For this review, take the finished solid that the model builds, in its own axes (mm). A direction names the side the tool comes from. Give positions to 0.01 mm unless a question says otherwise; leave off trailing zeros. Order: outer loops, then holes, each group sorted by start corner. A loop starts at its lowest first (then second) coordinate and runs counter-clockwise, first axis right, second up.
from build123d import *

# Parameters (mm, degrees)
BOSS_EXTRU_1_DEPTH      = 15
BOSS_EXTRU_2_DEPTH      = 2
BOSS_EXTRU_5_DEPTH      = 2
CONG_1_R                = 1
ENL_V_MAT_EXTRU_1_DEPTH = 2


with BuildPart() as part:
    # Esquisse1 → Boss.-Extru.1 (new body)
    with BuildSketch(Plane.XY):
        Polygon((-46.875775887, 92.331472327), (-146.875775887, -80.87360843), (53.124224113, -80.87360843), align=None)
        Polygon((44.463970075, -75.87360843), (-46.875775887, 82.331472327), (-138.21552185, -75.87360843), align=None, mode=Mode.SUBTRACT)
    extrude(amount=BOSS_EXTRU_1_DEPTH)

    # Esquisse2 → Boss.-Extru.2 (add)
    with BuildSketch(Plane(origin=(0, 0, 0), x_dir=(-1, 0, 0), z_dir=(0, 0, -1))):
        Polygon((-53.124224113, -80.87360843), (146.875775887, -80.87360843), (46.875775887, 92.331472327), align=None)
        Polygon((-42.731919267, -74.87360843), (136.483471042, -74.87360843), (46.875775887, 80.331472327), align=None, mode=Mode.SUBTRACT)
    extrude(amount=-BOSS_EXTRU_2_DEPTH)

    # Esquisse3 → Boss.-Extru.5 (add)
    # profile 1 of 3: a face of its own
    with BuildSketch(Plane.XY.offset(2)):
        Polygon((-76.884598102, 26.389185986), (-131.884598102, -68.87360843), (-134.307058992, -67.103952181), (-79.307058992, 28.158842235), align=None)
        Polygon((-78.199650653, 26.111448154), (-78.997792799, 26.694506994), (-132.992006441, -66.826214349), (-132.193864295, -67.409273189), align=None, mode=Mode.SUBTRACT)
    # profile 2 of 3: a face of its own
    with BuildSketch(Plane.XY.offset(2)):
        Polygon((16.217092488, -30.914062884), (18.960890201, -29.700978339), (-36.039109799, 65.561816078), (-38.782907512, 64.348731532), align=None)
        Polygon((16.634090745, -29.636325052), (17.538105586, -29.236643098), (-36.456108056, 64.284078245), (-37.360122897, 63.884396291), align=None, mode=Mode.SUBTRACT)
    # profile 3 of 3: a face of its own
    with BuildSketch(Plane.XY.offset(2)):
        Polygon((-85.155974471, -73.890867636), (-85.477311293, -76.87360843), (24.522688707, -76.87360843), (24.844025529, -73.890867636), align=None)
        Polygon((-84.257920177, -74.890867636), (-84.363792871, -75.87360843), (23.624634413, -75.87360843), (23.730507107, -74.890867636), align=None, mode=Mode.SUBTRACT)
    extrude(amount=BOSS_EXTRU_5_DEPTH)

    # Congé1
    # the kernel refuses this fillet: 1 mm, written as the material it takes off along each edge
    with BuildSketch(Plane(origin=(-40.032907512, 66.513795042, 2), x_dir=(0.8660254037844388, 0.49999999999999967, 0), z_dir=(0.49999999999999967, -0.8660254037844388, 0))) as cong_1_piece_1_section:
        with BuildLine():
            CenterArc((CONG_1_R, CONG_1_R), CONG_1_R, 180, 90)
            Line((0, CONG_1_R), (0, 0))
            Line((0, 0), (CONG_1_R, 0))
        make_face()
    cong_1_piece_1 = extrude(amount=115, mode=Mode.PRIVATE)
    cong_1_piece_1 = split(cong_1_piece_1, bisect_by=Plane(origin=(-10.431829018, 17.208704721, 2.226716308), z_dir=(-0.8660254037844386, -0.5000000000000001, 0)), keep=Keep.TOP, mode=Mode.PRIVATE)
    add(cong_1_piece_1, mode=Mode.SUBTRACT)
    with BuildSketch(Plane(origin=(-75.634598102, 28.554249495, 2), x_dir=(-0.8660254037844388, 0.4999999999999997, 0), z_dir=(-0.4999999999999997, -0.8660254037844388, 0))) as cong_1_piece_2_section:
        with BuildLine():
            CenterArc((CONG_1_R, -CONG_1_R), CONG_1_R, 90, 90)
            Line((0, -CONG_1_R), (0, 0))
            Line((0, 0), (CONG_1_R, 0))
        make_face()
    cong_1_piece_2 = extrude(amount=115, mode=Mode.PRIVATE)
    cong_1_piece_2 = split(cong_1_piece_2, bisect_by=Plane(origin=(-105.235676596, -20.750840825, 2.226716308), z_dir=(0.8660254037844387, -0.5000000000000001, 0)), keep=Keep.TOP, mode=Mode.PRIVATE)
    add(cong_1_piece_2, mode=Mode.SUBTRACT)
    with BuildSketch(Plane(origin=(27.344025529, -73.890867636, 2), x_dir=(0, -1, 0), z_dir=(-1, 0, 0))) as cong_1_piece_3_section:
        with BuildLine():
            CenterArc((CONG_1_R, CONG_1_R), CONG_1_R, 180, 90)
            Line((0, CONG_1_R), (0, 0))
            Line((0, 0), (CONG_1_R, 0))
        make_face()
    cong_1_piece_3 = extrude(amount=115, mode=Mode.PRIVATE)
    cong_1_piece_3 = split(cong_1_piece_3, bisect_by=Plane(origin=(-30.155974471, -74.87360843, 2.226716308), z_dir=(0, 1, 0)), keep=Keep.TOP, mode=Mode.PRIVATE)
    add(cong_1_piece_3, mode=Mode.SUBTRACT)

    # Esquisse3D1 → Enlèv. mat.-Extru.1 (cut)
    with BuildSketch(Plane(origin=(-138.21552185, -75.87360843, 0), x_dir=(1, 0, 0), z_dir=(0, 0, 1))):
        Polygon((0, 0), (182.679491924, 0), (91.339745962, 158.205080757), align=None)
        Polygon((1.732050808, 1), (180.947441117, 1), (91.339745962, 156.205080757), align=None, mode=Mode.SUBTRACT)
    extrude(amount=ENL_V_MAT_EXTRU_1_DEPTH, mode=Mode.SUBTRACT)


solid = part.part
1) Clearance check with flat-ended pins moving along their axes: pin 1 (0.8 mm diameter, centred on x = -25.5, z = 3.5, fed in from +Y); pin 2 (0.8 mm diameter, centred on x = -40, y = -75, fed in from -Z); pin 3 (1 mm diameter, centred on x = -33.5, y = -75, fed in from +Z). State where each tip first meets the part, or that it passes through.
Answer sheet:
pin 1: stops at y = 56
pin 2: stops at z = 2
pin 3: stops at z = 4
2) Tool access review of faces 4 (the face through (-48, -80.874, 7)), 5 (the face through (3.82, 4.52, 7.4)), 6 (the face through (-104.23, -20.38, 2.29)), 7 (the face through (-25, 42, 4)), 8 (the face through (-105.575, -21.304, 2.986)): name each direction out of +Z, -Z, +X, -X, +Y, -Y from which nothing blocks a thin tool from reaching the whole face with its end or side.
Answer sheet:
face 4: +Z, -Z, +X, -X, -Y
face 5: +Z, -Z, +X, +Y
face 6: -Z
face 7: +Z
face 8: +Z, -Z
3) We need section C-C on y = -58. Count the separate pieces of the cut face and the enclosed holes in it, then the cut area to 3 significant figures.
Answer sheet:
separate pieces: 3
enclosed holes: 0
area: 175 mm2
4) Draft analysis for pull direction X (two halves, no side actions). For faces 1 (the face through (-104, -20.58, 3.49)), 2 (the face through (-96.2, 6.9, 7.4)), 3 (the face through (-99, -7, 0)), state which applies: +X half, -X half, draft (parallel to the pull), parting line (faces both ways), or undercut.
Answer sheet:
face 1: undercut
face 2: -X half
face 3: draft
5) We need section B-B on z = 9.75. Give the boundary of the cut face in (x, y).
Answer sheet:
outline: (-146.88, -80.87) - (53.12, -80.87) - (-46.88, 92.33) - close; hole (-138.22, -75.87) - (44.46, -75.87) - (-46.88, 82.33) - close
6) We need section A-A on x = 37. Give the boundary of the cut face in (y, z).
Answer sheet:
outline: (-80.87, 0) - (-75.87, 0) - (-75.87, 15) - (-80.87, 15) - close; (-62.95, 0) - (-52.95, 0) - (-52.95, 15) - (-62.95, 15) - close
7) To check wall thickness, follow line 1 (Y direction, x = 19.5, z = 8); line 2 (Y direction, x = -104, z = 11.5); line 3 (X direction, y = 73, z = 10.5). State the ranges of each line that lie inside material, in increasing order.
Answer sheet:
line 1: y = -80.87 to -75.87, -32.63 to -22.63
line 2: y = -80.87 to -75.87, -16.61 to -6.61
line 3: x = -58.04 to -52.26, -41.49 to -35.71
